```python
from build123d import *

# Parameters (mm, degrees)
MAIN_BODY_DEPTH          = 2.6
SKETCH2_R                = 2.05
SKETCH2_R_2              = 1.5
SKETCH2_R_3              = 2.0499959
SCREW_HOLES_DEPTH        = 1
SCREW_HOLES_DEPTH_BACK   = 3.6
MAIN_LOWER_BODY_FILLET_R = 2
SKETCH5_W                = 17
SKETCH5_H                = 2.6
BOSS_EXTRUDE1_DEPTH      = 22.5
SKETCH6_W                = 2
SKETCH6_H                = 11
CUT_EXTRUDE1_DEPTH       = 22.5
FILLET2_R                = 2.5
SKETCH7_W                = 2.54
SKETCH7_H                = 1.27
CUT_EXTRUDE2_DEPTH       = 3.6


with BuildPart() as part:
    # Sketch1 → Main Body (new body)
    with BuildSketch(Plane(origin=(0, 0, 0), x_dir=(1, 0, 0), z_dir=(0, 1, 0))):
        with BuildLine():
            Line((11.7, -23.5), (32, -23.5))
            Line((32, -23.5), (32, 13.5))
            ThreePointArc((32, 13.5), (29.071067812, 20.571067812), (22, 23.5))
            Line((22, 23.5), (-22, 23.5))
            ThreePointArc((-22, 23.5), (-29.071067812, 20.571067812), (-32, 13.5))
            Line((-32, 13.5), (-32, -23.5))
            Line((-32, -23.5), (-12, -23.5))
            Line((-12, -23.5), (-12, -46))
            Line((-12, -46), (11.7, -46))
            Line((11.7, -46), (11.7, -23.5))
        make_face()
    extrude(amount=MAIN_BODY_DEPTH)

    # Sketch2 → Screw holes (cut, two sides)
    with BuildSketch(Plane(origin=(0, 2.6, 0), x_dir=(1, 0, 0), z_dir=(0, 1, 0))) as screw_holes_sk:
        with Locations((-20.1, 15.4999906)):
            Circle(SKETCH2_R)
        with Locations((20, 15.5)):
            Circle(SKETCH2_R)
        with Locations((-14.740009048, -4.250005346)):
            Circle(SKETCH2_R_2)
        with Locations((14.259990952, -4.250005346)):
            Circle(SKETCH2_R_2)
        with Locations((0.7, -28.9500094)):
            Circle(SKETCH2_R_3)
    extrude(amount=SCREW_HOLES_DEPTH, mode=Mode.SUBTRACT)
    extrude(screw_holes_sk.sketch, amount=-SCREW_HOLES_DEPTH_BACK, mode=Mode.SUBTRACT)

    # Main lower body Fillet
    main_lower_body_fillet_edges = [part.edges().sort_by_distance(p)[0] for p in [
        (11.7, 1.3, 46),
        (-12, 1.3, 46),
    ]]
    fillet(main_lower_body_fillet_edges, radius=MAIN_LOWER_BODY_FILLET_R)

    # Sketch5 → Boss-Extrude1 (add)
    with BuildSketch(Plane.XY.offset(23.5)):
        with Locations((-23.5, 1.3)):
            Rectangle(SKETCH5_W, SKETCH5_H)
        with Locations((23.5, 1.3)):
            Rectangle(SKETCH5_W, SKETCH5_H)
    extrude(amount=BOSS_EXTRUDE1_DEPTH)

    # Sketch6 → Cut-Extrude1 (cut)
    with BuildSketch(Plane(origin=(0, 2.6, 0), x_dir=(1, 0, 0), z_dir=(0, 1, 0))):
        with Locations((-21, -40.5)):
            Rectangle(SKETCH6_W, SKETCH6_H)
        with Locations((21, -40.5)):
            Rectangle(SKETCH6_W, SKETCH6_H)
    extrude(amount=-CUT_EXTRUDE1_DEPTH, mode=Mode.SUBTRACT)

    # Fillet2
    fillet2_edges = [part.edges().sort_by_distance(p)[0] for p in [
        (-32, 1.3, 46),
        (-15, 1.3, 46),
        (32, 1.3, 46),
        (15, 1.3, 46),
    ]]
    fillet(fillet2_edges, radius=FILLET2_R)

    # Sketch7 → Cut-Extrude2 (cut, through all)
    with BuildSketch(Plane(origin=(0, 2.6, 0), x_dir=(1, 0, 0), z_dir=(0, 1, 0))):
        with Locations((-30.73, -24.135)):
            Rectangle(SKETCH7_W, SKETCH7_H)
        with Locations((30.73, -24.135)):
            Rectangle(SKETCH7_W, SKETCH7_H)
        with Locations((-16.27, -24.135)):
            Rectangle(SKETCH7_W, SKETCH7_H)
        with Locations((16.27, -24.135)):
            Rectangle(SKETCH7_W, SKETCH7_H)
    extrude(amount=-CUT_EXTRUDE2_DEPTH, mode=Mode.SUBTRACT)


solid = part.part
```
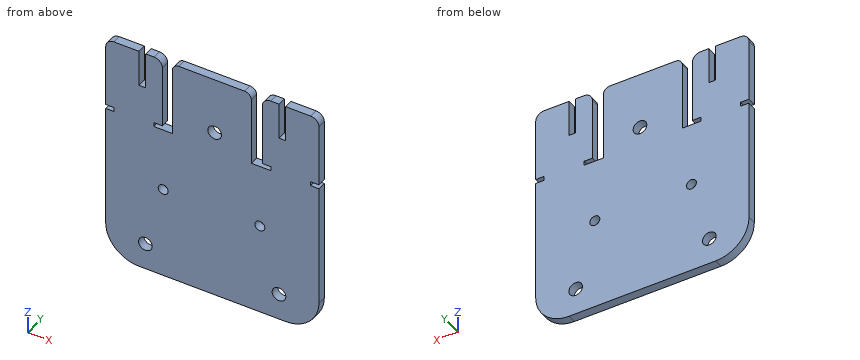
Source: CAD feature listing. Evaluate the final solid. Frame: model axes, mm. Round coordinates to 2 decimals unless told otherwise and drop trailing zeros. Loops run counter-clockwise (first coordinate to the right, second up) from the corner with the lowest first, then second, coordinate; pieces in that order, holes last. Notation, with made-up numbers: (-5, -36.75) - (25, -36.75) arc R33 ccw to (25, 0.25) - close; hole circle Ø10 at (-10.5, -11). An arc over 180 degrees is marked (long way). Use CSV: the item, a comma, the result in double quotes.
Q1. Pin query (flat end, axial travel): pin 1 Ø0.6 at (y, z) = (0.5, 24) entering from -X; pin 2 Ø0.6 at (y, z) = (1, 24) entering from +X; pin 3 Ø1.3 at (x, y) = (-31, 1.5) entering from +Z. Return the tip coordinate at first contact, or that it passes through.
Reported:
pin 1,"x = -29.46"
pin 2,"x = 29.46"
pin 3,"z = 45.85"
Q2. Section query A-A, the plane x = 0.7. Output: boundary loops of the cut face in (y, z).
Reported:
outline,"(0, -23.5) - (2.6, -23.5) - (2.6, 26.9) - (0, 26.9) - close; (0, 31) - (2.6, 31) - (2.6, 46) - (0, 46) - close"
Q3. Section query B-B, the plane y = 1.8. Give the number of separate pieces and of enclosed holes in the cut face, then the cut area to 3 significant figures.
Reported:
separate pieces,"1"
enclosed holes,"5"
area,"4,150 mm^2"
Q4. Ray query, line 1 along Z through (x, y) = (0.7, 1.4); line 2 along Z through (x, y) = (-20.1, 1.8); line 3 along X through (y, z) = (0.4, -15.5). Return the intervals inside material, ascending.
Reported:
line 1,"-23.5 to 26.9, 31 to 46"
line 2,"-23.5 to -17.55, -13.45 to 35"
line 3,"-31.8 to -22.15, -18.05 to 17.95, 22.05 to 31.8"
